Solid Edge part; units mm, degrees
sketch "Sketch1" plane through (0, 0, 0) normal (0, -1, 0) x (1, 0, 0)
  line L0 (0, 0) -> (57.7787, 5.175)
  line L1 (57.7787, 5.175) -> (57.7787, -5.175)
  line L2 (57.7787, -5.175) -> (0, 0)
extrude "Protrusion1" add sketch "Sketch1" against normal blind 1.6
sketch "Sketch2" plane through (28.8062, 0, 0) normal (0, -1, 0) x (0.996013, 0, -0.0892088)
  circle A0 centre (23.6777, 2.1207) radius 1.5
extrude "Cutout1" cut sketch "Sketch2" against normal up to next
sketch "Sketch3" plane through (28.8062, 0, 0) normal (0, -1, 0) x (0.996013, 0, -0.0892088)
  circle A0 centre (23.6777, 2.1207) radius 1.5
  line L0 (29.3186, -2.5698) -> (-28.6914, -2.5698)
  line L1 (28.3953, 7.739) -> (29.3186, -2.5698)
  line L2 (1.8202, 2.94) -> (28.3953, 7.739)
  line L3 (0.5673, 9.8778) -> (1.8202, 2.94)
  arc A1 (-3.369, 9.167) -> (0.5673, 9.8778) centre (-1.4008, 9.5224) cw
  line L4 (-2.1162, 2.2292) -> (-3.369, 9.167)
  line L5 (-28.6914, -2.5698) -> (-2.1162, 2.2292)
  circle A2 centre (-0.5656, 4.8972) radius 0.75
  circle A3 centre (-0.9832, 7.2098) radius 0.75
  circle A4 centre (-1.4008, 9.5224) radius 0.75
extrude "Protrusion2" add sketch "Sketch3" against normal up to vertex (1.6 mm away)
properties material "Wood, balsa"
Geometry check sheet. Reference: the model listing, model coordinates, mm. A direction names the side the tool comes from. Give positions to 0.01 mm unless a question says otherwise; leave off trailing zeros. Order: outer loops, then holes, each group sorted by start corner. A loop starts at its lowest first (then second) coordinate and runs counter-clockwise, first axis right, second up. Notation, with made-up numbers: (-12.75, 87) - (-1.75, 87) arc R15 cw to (-1.75, 107) - close; hole circle Ø3 at (17.5, 71). An arc over 180 degrees is marked (long way). Answer in a Markdown table with one row per item. Add a question column.
Q1. Tool access check on faces 1 (the flat face through (57.779, 1, 0)), 2 (the flat face through (30.563, 0.789, 6.326)), 3 (the flat face through (26.587, 0.789, 5.871)). Record the directions out of +Z, -Z, +X, -X, +Y, -Y that give a thin tool (end or side, any length) a straight path to the whole face; none if there is none.
Q2. Cross-section at C-C, the plane z = -4. Enter the section's corners in (x, y).
Q3. Cross-section at B-B, the plane x = 11.5. Enter the section's corners in (y, z), then the cut area to 3 significant figures.
Q4. Mould release check, pull along Z, two halves, no side actions. Record for faces 4 (the cylindrical face through (51.092, 0.789, 0.199)), 5 (the flat face through (29.294, 0.789, -2.624)), 6 (the flat face through (38, 1.6, 1)): pulls with the +Z half, pulls with the -Z half, needs draft (parallel to the pull), parting line crosses it, or undercut.
Q5. Material ranges on probe 1 along X at (y, z) = (0.8, 7.75); probe 2 along Z at (x, y) = (52, 0.4); probe 3 along Z at (x, y) = (7, 1.3), recorded low to high. Write a range as from..to.
Q6. Gauge pin test, flat end, axial feed: pin 1 (1.4 mm diameter, centred on x = 28.26, z = 9.61, fed in from +Y). Record the tip position at first contact, or that the pin passes through.
Check values:
| question | item | result |
|---|---|---|
| 1 | face 1 | +Z, -Z, +X, +Y, -Y |
| 1 | face 2 | +Z, +Y, -Y |
| 1 | face 3 | -X, +Y, -Y |
| 2 | outline | (44.66, 0) - (57.78, 0) - (57.78, 1.6) - (44.66, 1.6) - close |
| 3 | outline | (0, -1.03) - (1.6, -1.03) - (1.6, 1.03) - (0, 1.03) - close |
| 3 | area | 3.30 mm^2 |
| 4 | face 4 | undercut |
| 4 | face 5 | pulls with the -Z half |
| 4 | face 6 | needs draft |
| 5 | probe 1 | x = 26.42..27.89, 29.05..30.44 |
| 5 | probe 2 | z = -4.66..-1.38, 1.38..4.66 |
| 5 | probe 3 | z = -0.63..0.63 |
| 6 | pin 1 | passes through |
